For this review, take the finished solid that the model builds, in its own axes (mm). Face numbers are marked on the shaded views. A direction names the side the tool comes from. Round coordinates to 2 decimals unless told otherwise and drop trailing zeros. Order: outer loops, then holes, each group sorted by start corner. A loop starts at its lowest first (then second) coordinate and runs counter-clockwise, first axis right, second up. Notation, with made-up numbers: (27, 58) - (62, 58) arc R19 ccw to (62, 66) - close; hole circle Ø4 at (85, -21.75). An arc over 180 degrees is marked (long way). One line per question, with ' | ' between items.
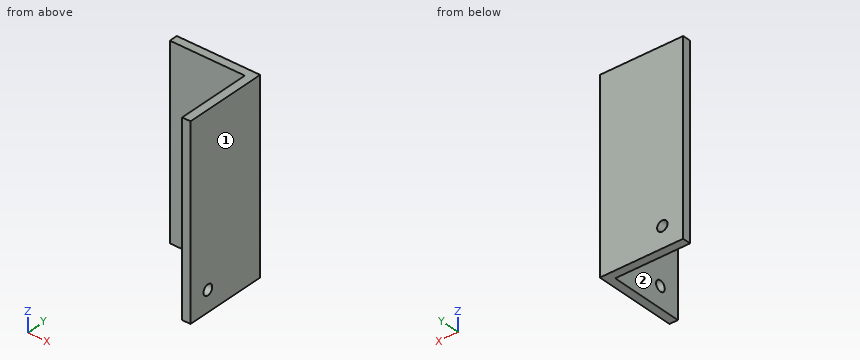
```python
from build123d import *

# Parameters (mm, degrees)
F0_W     = 25.4
F0_H     = 57.15
F1_DEPTH = 25.4
F2_T     = -2.54
F4_D     = 3.175
F6_D     = 3.175


with BuildPart() as f1:
    # F0 (on Front) → F1 (new body)
    with BuildSketch(Plane.XZ):
        with Locations((27.139076, -1.29187)):
            Rectangle(F0_W, F0_H)
    extrude(amount=F1_DEPTH)

    # F2
    f2_openings = [f1.faces().sort_by_distance(p)[0] for p in [
        (27.139076, -12.7, 27.28313),
        (27.139076, -25.4, -1.29187),
        (14.439076, -12.7, -1.29187),
        (27.139076, -12.7, -29.86687),
    ]]
    offset(amount=F2_T, openings=f2_openings)

    # F4 (through all)
    with Locations(Plane.YZ.offset(39.839076)):
        with Locations((-19.05, -23.51687)):
            Hole(F4_D / 2)

    # F6 (through all)
    with Locations(Plane(origin=(0, 0, 0), x_dir=(-1, 0, 0), z_dir=(0, 1, 0))):
        with Locations((-20.789076, -23.51687)):
            Hole(F6_D / 2)


solid = f1.part
```
(1) We need section C-C on y = -12.75. State the section outline as (x, z) points, plus the area to 3 significant figures.
Output values:
outline: (37.3, -29.87) - (39.84, -29.87) - (39.84, 27.28) - (37.3, 27.28) - close | area: 145 mm^2
(2) We need section A-A on y = -19.05. State the section outline as (x, z) points, plus the area to 3 significant figures.
Output values:
outline: (37.3, -29.87) - (39.84, -29.87) - (39.84, -25.1) - (37.3, -25.1) - close; (37.3, -21.93) - (39.84, -21.93) - (39.84, 27.28) - (37.3, 27.28) - close | area: 137 mm^2
(3) We need section D-D on x = 33.5. State the section outline as (y, z) points, plus the area to 3 significant figures.
Output values:
outline: (-2.54, -29.87) - (0, -29.87) - (0, 27.28) - (-2.54, 27.28) - close | area: 145 mm^2
(4) For probe 1 along Z at (x, y) = (38.2, -19.05); probe 2 along X at (y, z) = (-10, 21.5); probe 3 along Y at (x, z) = (18.5, -23.5), list the stretches that pass through material, from the lowest coordinate up. Write a range as [from, to].
Output values:
probe 1: [-29.87, -25.1], [-21.93, 27.28] | probe 2: [37.3, 39.84] | probe 3: [-2.54, 0]
(5) For the marked faces 1 and 2, list the 3-axis set-ups (+Z, -Z, +X, -X, +Y, -Y) from which the entire face can be reached by the end or side of a thin tool; tool diameter is ignored.
Output values:
face 1: +Z, -Z, +X, +Y, -Y | face 2: +Z, -Z, -X, -Y
(6) Insertion check: pin 1 (4 mm diameter, centred on x = 20.79, z = -23.52, fed in from -Y); pin 2 (7 mm diameter, centred on y = -13.5, z = 10.5, fed in from -X); pin 3 (12 mm diameter, centred on x = 35, y = -12, fed in from +Z). Each pin has a flat end and moves straight along its axis. Give the tip position at first contact, or say it passes through.
Output values:
pin 1: y = -2.54 | pin 2: x = 37.3 | pin 3: z = 27.28
(7) We need section B-B on z = 0.5. State the section outline as (x, y) points.
Output values:
outline: (14.44, -2.54) - (37.3, -2.54) - (37.3, -25.4) - (39.84, -25.4) - (39.84, 0) - (14.44, 0) - close
